from build123d import *

# Parameters (mm, degrees)
SKETCH1_R           = 93.17284
SKETCH1_W           = 100
SKETCH1_H           = 40
BOSS_EXTRUDE1_DEPTH = 540
SKETCH2_OUTSIDE_W   = 308.52
SKETCH2_OUTSIDE_H   = 308.52
SKETCH2_OUTSIDE_R   = 83.17284
CUT_EXTRUDE2_DEPTH  = 541


with BuildPart() as part:
    # Sketch1 → Boss-Extrude1 (new body)
    with BuildSketch(Plane(origin=(0, 0, 0), x_dir=(0, 0, -1), z_dir=(1, 0, 0))):
        Circle(SKETCH1_R)
        with Locations((0, -30)):
            Rectangle(SKETCH1_W, SKETCH1_H, mode=Mode.SUBTRACT)
    extrude(amount=BOSS_EXTRUDE1_DEPTH)

    # Sketch2 outside → Cut-Extrude2 (cut, through all)
    with BuildSketch(Plane(origin=(540, 0, 0), x_dir=(0, 0, -1), z_dir=(1, 0, 0))):
        Rectangle(SKETCH2_OUTSIDE_W, SKETCH2_OUTSIDE_H)
        Circle(SKETCH2_OUTSIDE_R, mode=Mode.SUBTRACT)
    extrude(amount=-CUT_EXTRUDE2_DEPTH, mode=Mode.SUBTRACT)


solid = part.part
The listing builds one solid part. Answer for the finished solid, in the listing's coordinates (mm). A direction names the side the tool comes from. Give positions to 0.01 mm unless a question says otherwise; leave off trailing zeros. Order: outer loops, then holes, each group sorted by start corner. A loop starts at its lowest first (then second) coordinate and runs counter-clockwise, first axis right, second up. Notation, with made-up numbers: (80.25, 12.5) - (111.25, 12.5) arc R19 cw to (111.25, 20.5) - close; hole circle Ø9 at (-25.5, -21). An arc over 180 degrees is marked (long way). One line per item, written item: value. Start each with the question number.
1) Find the intervals of material crossed by L1, parallel to Y at x = 480, z = 32; L2, parallel to Y at x = 501.5, z = 24; L3, parallel to Z at x = 432.5, y = -5, in increasing order.
2) A cutting plane is placed at C-C on y = -29. Give the vertices of the cut face in (x, z), then the cut area to 3 significant figures.
3) A tool of negligible diameter and unlimited length cuts with its end or side. For faces 1 (the face through (266, -30, 50)), 2 (the face through (0, 1, 1)), from which of +Z, -Z, +X, -X, +Y, -Y can it reach the whole face along a straight path? Write none if from no direction.
4) A cutting plane is placed at A-A on z = 0. Give the vertices of the cut face in (x, y), then the cut area to 3 significant figures.
5) A cutting plane is placed at D-D on z = 71.5. Give the vertices of the cut face in (x, y), then the cut area to 3 significant figures.
6) The mould has two halves that part along Z. Classify faces 3 (the face through (273.8, -81.2, 18)), 4 (the face through (540, 1, 1)), 5 (the face through (266, -50, 1)): released by +Z, released by -Z, zero draft, split by the parting line, or undercut.
7) Given pin 1 Ø8 at (x, y) = (407.5, 62.5) entering from +Z; pin 2 Ø3 at (x, y) = (80, -28) entering from -Z; pin 3 Ø20 at (x, y) = (231.5, -27.5) entering from +Z, each flat-ended and moving along its own axis, determine where each tip first touches the part or whether it passes through.
8) A cutting plane is placed at B-B on x = 101.5. Give the vertices of the cut face in (y, z).
Answer sheet:
1. L1: y = -76.77 to -50, -10 to 76.77
1. L2: y = -79.63 to -50, -10 to 79.63
1. L3: z = -83.02 to 83.02
2. outline: (0, -77.95) - (540, -77.95) - (540, -50) - (0, -50) - close; (0, 50) - (540, 50) - (540, 77.95) - (0, 77.95) - close
2. area: 30,200 mm2
3. face 1: +X, -X
3. face 2: +Z, -Z, -X, +Y, -Y
4. outline: (0, -83.17) - (540, -83.17) - (540, -50) - (0, -50) - close; (0, -10) - (540, -10) - (540, 83.17) - (0, 83.17) - close
4. area: 68,200 mm2
5. outline: (0, -42.49) - (540, -42.49) - (540, 42.49) - (0, 42.49) - close
5. area: 45,900 mm2
6. face 3: split by the parting line
6. face 4: zero draft
6. face 5: undercut
7. pin 1: stops at z = 59.12
7. pin 2: stops at z = -78.84
7. pin 3: stops at z = 81.31
8. outline: circle Ø166.35 at (0, 0); hole (-50, -50) - (-10, -50) - (-10, 50) - (-50, 50) - close
